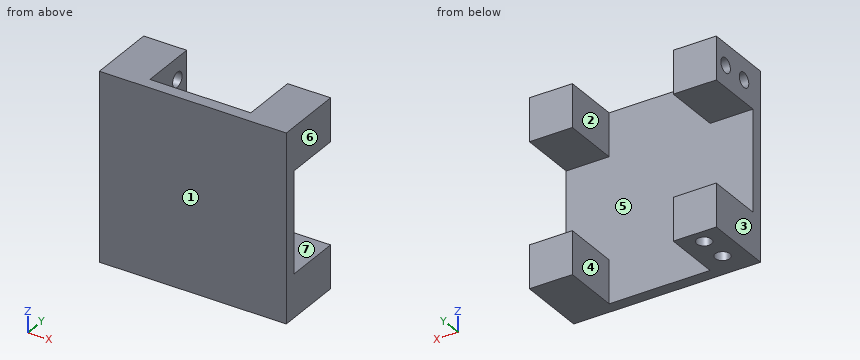
Autodesk Inventor part; units mm, degrees
ref_plane "YZ Plane" through (0, 0, 0) normal (1, 0, 0) x (0, 1, 0)
ref_plane "XZ Plane" through (0, 0, 0) normal (0, 1, 0) x (-1, 0, 0)
ref_plane "XY Plane" through (0, 0, 0) normal (0, 0, 1) x (1, 0, 0)
sketch "Sketch1" plane through (0, 0, 0) normal (0, 0, 1) x (1, 0, 0)
  line L0 (0, 0) -> (50.8, 0)
  line L1 (50.8, 0) -> (50.8, 3.175)
  line L2 (50.8, 3.175) -> (0, 3.175)
  line L3 (0, 3.175) -> (0, 0)
  line L4 (0, 3.175) -> (11.684, 3.175)
  line L5 (11.684, 3.175) -> (11.684, 18.669)
  line L6 (11.684, 18.669) -> (0, 18.669)
  line L7 (0, 18.669) -> (0, 3.175)
  line L8 (50.8, 3.175) -> (39.116, 3.175)
  line L9 (39.116, 3.175) -> (39.116, 18.669)
  line L10 (39.116, 18.669) -> (50.8, 18.669)
  line L11 (50.8, 18.669) -> (50.8, 3.175)
  dimension "d0" = 50.8
  dimension "d1" = 3.175
  dimension "d2" = 11.684
  dimension "d3" = 15.494
  dimension "d4" = 11.684
  dimension "d5" = 15.494
extrude "Extrusion1" add sketch "Sketch1" against normal blind 50.8
sketch "Sketch2" plane through (50.8, 0, 0) normal (1, 0, 0) x (0, 0, -1)
  line L0 (0, 3.175) -> (0, 18.669)
  line L1 (0, 3.175) -> (11.684, 3.175)
  line L2 (11.684, 3.175) -> (11.684, 18.669)
  line L3 (11.684, 18.669) -> (0, 18.669)
  line L4 (0, 18.669) -> (0, 3.175)
  line L5 (0, 18.669) -> (50.8, 18.669)
  line L6 (0, 3.175) -> (50.8, 3.175)
  line L7 (50.8, 18.669) -> (39.116, 18.669)
  line L8 (39.116, 18.669) -> (39.116, 3.175)
  line L9 (39.116, 3.175) -> (50.8, 3.175)
  line L10 (50.8, 3.175) -> (50.8, 18.669)
  line L11 (11.684, 3.175) -> (39.116, 3.175)
  point P0 (0, 0)
  dimension "d8" = 11.684
  dimension "d9" = 15.494
  dimension "d10" = 11.684
extrude "Extrusion2" cut sketch "Sketch2" against normal blind 50.8 contours L2 L5 L8 L6
sketch "Sketch3" plane through (0, 0, 0) normal (-1, 0, 0) x (0, 0, 1)
  line L0 (0, 3.175) -> (-11.684, 3.175)
  circle A0 centre (-5.842, 6.985) radius 2
  line L1 (0, 3.175) -> (0, 18.669)
  circle A1 centre (-5.842, 14.732) radius 2
  point P0 (0, 0)
  dimension "d14" = 4
  dimension "d16" = 4
extrude "Extrusion3" cut sketch "Sketch3" against normal up to surface (11.684 mm away)
sketch "Sketch4" plane through (0, 0, -50.8) normal (0, 0, -1) x (-1, 0, 0)
  line L0 (-11.684, 3.175) -> (0, 3.175)
  circle A0 centre (-5.842, 6.985) radius 2
  line L1 (-11.684, 3.175) -> (-11.684, 18.669)
  line L2 (0, 18.669) -> (0, 3.175)
  circle A1 centre (-5.842, 14.732) radius 2
  point P0 (0, 0)
  dimension "d20" = 4
  dimension "d22" = 4
extrude "Extrusion4" cut sketch "Sketch4" against normal up to surface (11.684 mm away)
properties part number "Ruler square"
Check sheet for the modelled part. Datum: model origin and axes. Units: mm. Face numbers are marked on the shaded views. A direction names the side the tool comes from. Round coordinates to 2 decimals unless told otherwise and drop trailing zeros. Write each loop counter-clockwise with the first axis right and the second up, starting at its lowest first coordinate (ties: lowest second). Pieces come first, ordered by that corner, then holes. Notation, with made-up numbers: (84, 21.5) -> (134, 21.5) arc R20 ccw to (134, 36.5) -> close; hole circle Ø3 at (-4, 3.25). An arc over 180 degrees is marked (long way). Answer as CSV lines item,"result". Start each with the question number.
1) Section check B-B on z = -46. Enter the section's corners in (x, y) (3 decimals).
2) Material ranges on line 1 (Z direction, x = 42, y = 8.5); line 2 (X direction, y = 8.5, z = -3); line 3 (Z direction, x = 11, y = 13), recorded low to high. Write a range as from..to.
3) Section check A-A on y = 11.5. Enter the section's corners in (x, z), and give its area (3 significant figures).
4) Tool access check on the marked faces 5, 6 and 7. Record the directions out of +Z, -Z, +X, -X, +Y, -Y that give a thin tool (end or side, any length) a straight path to the whole face; none if there is none.
5) Go/stop test with a flat-tipped pin: P1, Ø1.5, axis at x = 5.5, z = -20, coming from the +Y side (3 decimals). Record where the tip stops, or that it passes through.
6) Section check C-C on x = 11. Enter the section's corners in (y, z) (3 decimals), and give its area (3 significant figures).
7) Section check D-D on y = 15.75. Enter the section's corners in (x, z).
8) Release check for a two-part mould opening along X. For the marked faces 1, 2, 3 and 4 record: pulls with the +X half, pulls with the -X half, needs draft (parallel to the pull), parting line crosses it, or undercut.
Found:
1,outline,"(0, 0) -> (50.8, 0) -> (50.8, 18.669) -> (39.116, 18.669) -> (39.116, 3.175) -> (11.684, 3.175) -> (11.684, 18.669) -> (0, 18.669) -> close; hole circle Ø4 at (5.842, 6.985); hole circle Ø4 at (5.842, 14.732)"
2,line 1,"z = -50.8..-39.12, -11.68..0"
2,line 2,"x = 0..11.68, 39.12..50.8"
2,line 3,"z = -50.8..-39.12, -11.68..-6.84, -4.84..0"
3,outline,"(0, -50.8) -> (11.68, -50.8) -> (11.68, -39.12) -> (0, -39.12) -> close; (0, -11.68) -> (11.68, -11.68) -> (11.68, 0) -> (0, 0) -> close; (39.12, -50.8) -> (50.8, -50.8) -> (50.8, -39.12) -> (39.12, -39.12) -> close; (39.12, -11.68) -> (50.8, -11.68) -> (50.8, 0) -> (39.12, 0) -> close"
3,area,"546 mm^2"
4,face 5,"+Y"
4,face 6,"+Z, -Z, +X, +Y, -Y"
4,face 7,"+X, -X, +Y"
5,P1,"stops at y = 3.175"
6,outline,"(0, -50.8) -> (18.669, -50.8) -> (18.669, -39.116) -> (3.175, -39.116) -> (3.175, -11.684) -> (18.669, -11.684) -> (18.669, 0) -> (0, 0) -> close; hole circle Ø4 at (6.985, -5.842); hole circle Ø4 at (14.732, -5.842)"
6,area,"498 mm^2"
7,outline,"(0, -50.8) -> (4.12, -50.8) -> (4.12, -39.12) -> (0, -39.12) -> close; (0, -11.68) -> (11.68, -11.68) -> (11.68, -7.56) -> (0, -7.56) -> close; (0, -4.12) -> (11.68, -4.12) -> (11.68, 0) -> (0, 0) -> close; (7.56, -50.8) -> (11.68, -50.8) -> (11.68, -39.12) -> (7.56, -39.12) -> close; (39.12, -50.8) -> (50.8, -50.8) -> (50.8, -39.12) -> (39.12, -39.12) -> close; (39.12, -11.68) -> (50.8, -11.68) -> (50.8, 0) -> (39.12, 0) -> close"
8,face 1,"needs draft"
8,face 2,"undercut"
8,face 3,"pulls with the -X half"
8,face 4,"undercut"
